from build123d import *

# Parameters (mm, degrees)
SKETCH1_W            = 84.3
SKETCH1_H            = 84.3
SKETCH1_W_2          = 80.3
SKETCH1_H_2          = 80.3
BOSS_EXTRUDE1_DEPTH  = 10
BOSS_EXTRUDE2_DEPTH  = 80
MIRROR2_COPY_1_DEPTH = 80
FILLET1_R            = 2


with BuildPart() as part:
    # Sketch1 → Boss-Extrude1 (new body)
    with BuildSketch(Plane(origin=(0, 0, 0), x_dir=(1, 0, 0), z_dir=(0, 1, 0))):
        Rectangle(SKETCH1_W, SKETCH1_H)
        Rectangle(SKETCH1_W_2, SKETCH1_H_2, mode=Mode.SUBTRACT)
    extrude(amount=BOSS_EXTRUDE1_DEPTH)

    # Sketch2 → Boss-Extrude2 (add)
    with BuildSketch(Plane.XZ):
        Polygon((-42.15, 30.15), (-40.15, 30.15), (-40.15, 40.15), (-30.15, 40.15), (-30.15, 42.15), (-42.15, 42.15), align=None)
    boss_extrude2 = extrude(amount=BOSS_EXTRUDE2_DEPTH)

    # Mirror1: Boss-Extrude2 across plane
    add(boss_extrude2.mirror(Plane(origin=(0, 0, 0), x_dir=(0, 0, 1), z_dir=(1, 0, 0))))

    # Mirror2: Boss-Extrude2 across plane
    add(boss_extrude2.mirror(Plane.XY))

    # Mirror2 copy 1 sketch → Mirror2 copy 1 (add)
    with BuildSketch(Plane(origin=(0, 0, 0), x_dir=(-1, 0, 0), z_dir=(0, -1, 0))):
        Polygon((-42.15, 30.15), (-40.15, 30.15), (-40.15, 40.15), (-30.15, 40.15), (-30.15, 42.15), (-42.15, 42.15), align=None)
    extrude(amount=MIRROR2_COPY_1_DEPTH)

    # Fillet1
    fillet1_edges = [part.edges().sort_by_distance(p)[0] for p in [
        (40.15, -35, 40.15),
        (40.15, -35, -40.15),
        (-40.15, -35, -40.15),
        (-40.15, -35, 40.15),
        (-41.15, 0, 30.15),
        (-30.15, 0, 41.15),
        (30.15, 0, 41.15),
        (41.15, 0, 30.15),
        (-30.15, 0, -41.15),
        (-41.15, 0, -30.15),
        (-42.15, -35, -42.15),
        (42.15, -35, -42.15),
        (42.15, -35, 42.15),
        (-42.15, -35, 42.15),
        (41.15, 0, -30.15),
        (30.15, 0, -41.15),
    ]]
    fillet(fillet1_edges, radius=FILLET1_R)


solid = part.part
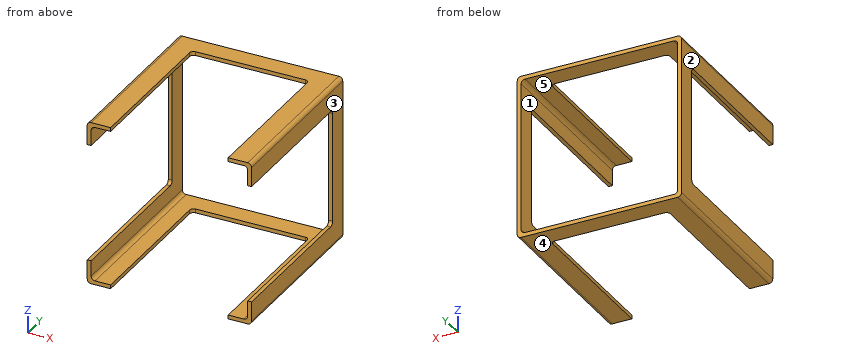
Geometry: final body of the model. Coordinates: model frame, mm. Face numbers are marked on the shaded views. A direction names the side the tool comes from. Round coordinates to 2 decimals unless told otherwise and drop trailing zeros. Loops run counter-clockwise (first coordinate to the right, second up) from the corner with the lowest first, then second, coordinate; pieces in that order, holes last. Notation, with made-up numbers: M 43,52 L 91,52 A25 ccw 91,87 Z; hole C 4,45.25 d3. An arc over 180 degrees is marked long. One line per question, with ' | ' between items.
(1) Material intervals for line 1 along Z through (x, y) = (-34, -10); line 2 along X through (y, z) = (-28.5, -38.5), sorted ascending. Write a range as from..to.
Check result:
line 1: z = -42.15..-40.15, 40.15..42.15 | line 2: x = -42.15..-40.12, 40.12..42.15
(2) Contact query for flat-ended pins moving along their axis: P1, Ø0.6, axis at x = -41, y = -36.5, coming from the +Z side; P2, Ø1.6, axis at y = -28, z = -41.5, coming from the -X side; P3, Ø0.6, axis at x = -41.5, y = -38.5, coming from the -Z side; P4, Ø23, axis at x = -16.5, y = -47.5, coming from the -Z side. Output: stop coordinate, or through.
Check result:
P1: stops at z = 42.07 | P2: stops at x = -42.07 | P3: stops at z = -41.85 | P4: passes through
(3) Cut plane A-A on x = -34.5. Return the cut outline in (y, z).
Check result:
outline: M -80,-42.15 L 10,-42.15 L 10,-40.15 L -80,-40.15 Z; M -80,40.15 L 10,40.15 L 10,42.15 L -80,42.15 Z
(4) Pull-direction query (X, two-part tool) for the marked faces 1, 2 and 3; classes: +X half, -X half, draft (parallel to the pull), parting line (faces both ways), or undercut.
Check result:
face 1: undercut | face 2: -X half | face 3: +X half
(5) Access query for the marked faces 4 and 5. Directions: +Z, -Z, +X, -X, +Y, -Y. A direction counts if a zero-diameter tool reaches every point of the face in a straight line with its end or side. Return the directions, or none.
Check result:
face 4: -Z, +X, -X, +Y, -Y | face 5: +Y, -Y
(6) Cut plane B-B on z = 1. Return the cut outline in (x, y), plus the area to 3 significant figures.
Check result:
outline: M -42.15,0 L -40.15,0 L -40.15,10 L -42.15,10 Z; M 40.15,0 L 42.15,0 L 42.15,10 L 40.15,10 Z | area: 40.0 mm2
(7) Cut plane C-C on y = -64.5. Give the number of separate pieces and of enclosed holes in the cut face, plus the area to 3 significant figures.
Check result:
separate pieces: 4 | enclosed holes: 0 | area: 176 mm2
